```python
from build123d import *

# Parameters (mm, degrees)
SKETCH_1_W               = 15
SKETCH_1_H               = 15
SKETCH_1_W_2             = 6
SKETCH_1_H_2             = 6
SKETCH_1_W_3             = 2
SKETCH_1_H_3             = 2.75
SKETCH_1_W_4             = 2.75
SKETCH_1_H_4             = 2
EXTRUDE_1_DEPTH          = 10
SKETCH_2_W               = 2
SKETCH_2_H               = 4
CUT_EXTRUDE_1_DEPTH      = 2.75
SKETCH_3_W               = 4
SKETCH_3_H               = 2
CUT_EXTRUDE_2_DEPTH      = 2.75
SKETCH_4_W               = 2
SKETCH_4_H               = 4
CUT_EXTRUDE_3_DEPTH      = 2.75
SKETCH_5_W               = 4
SKETCH_5_H               = 2
CUT_EXTRUDE_4_DEPTH      = 2.75
SKETCH_6_W               = 5.5
SKETCH_6_H               = 3
CUT_EXTRUDE_5_DEPTH      = 18.75
SKETCH_7_W               = 3
SKETCH_7_H               = 5.5
CUT_EXTRUDE_6_DEPTH      = 18.75
SKETCH_8_W               = 8
SKETCH_8_H               = 13
CUT_EXTRUDE_7_DEPTH      = 6
CUT_EXTRUDE_7_DEPTH_BACK = 0.75
SKETCH_9_W               = 8
SKETCH_9_H               = 13
CUT_EXTRUDE_8_DEPTH      = 6
SKETCH_10_W              = 8
SKETCH_10_H              = 13
CUT_EXTRUDE_9_DEPTH      = 6


with BuildPart() as part:
    # ｽｹｯﾁ1 → ﾎﾞｽ - 押し出し1 (new body)
    with BuildSketch(Plane.XY):
        with Locations((-13.66786655, 0.754091784)):
            Rectangle(SKETCH_1_W, SKETCH_1_H)
        with Locations((-17.16786655, -2.745908216)):
            Rectangle(SKETCH_1_W_2, SKETCH_1_H_2, mode=Mode.SUBTRACT)
        with Locations((-10.16786655, -2.745908216)):
            Rectangle(SKETCH_1_W_2, SKETCH_1_H_2, mode=Mode.SUBTRACT)
        with Locations((-10.16786655, 4.254091784)):
            Rectangle(SKETCH_1_W_2, SKETCH_1_H_2, mode=Mode.SUBTRACT)
        with Locations((-17.16786655, 4.254091784)):
            Rectangle(SKETCH_1_W_2, SKETCH_1_H_2, mode=Mode.SUBTRACT)
        with Locations((-13.66786655, 9.629091784)):
            Rectangle(SKETCH_1_W_3, SKETCH_1_H_3)
        with Locations((-22.54286655, 0.754091784)):
            Rectangle(SKETCH_1_W_4, SKETCH_1_H_4)
        with Locations((-4.79286655, 0.754091784)):
            Rectangle(SKETCH_1_W_4, SKETCH_1_H_4)
        with Locations((-13.66786655, -8.120908216)):
            Rectangle(SKETCH_1_W_3, SKETCH_1_H_3)
    extrude(amount=EXTRUDE_1_DEPTH)

    # ｽｹｯﾁ2 → ｶｯﾄ - 押し出し1 (cut)
    with BuildSketch(Plane(origin=(0, 11.004091784, 0), x_dir=(1, 0, 0), z_dir=(0, 1, 0))):
        with Locations((-13.66786655, -2)):
            Rectangle(SKETCH_2_W, SKETCH_2_H)
        with Locations((-13.66786655, -8)):
            Rectangle(SKETCH_2_W, SKETCH_2_H)
    extrude(amount=-CUT_EXTRUDE_1_DEPTH, mode=Mode.SUBTRACT)

    # ｽｹｯﾁ3 → ｶｯﾄ - 押し出し2 (cut)
    with BuildSketch(Plane(origin=(-3.41786655, 0, 0), x_dir=(0, 0, -1), z_dir=(1, 0, 0))):
        with Locations((-8, 0.754091784)):
            Rectangle(SKETCH_3_W, SKETCH_3_H)
        with Locations((-2, 0.754091784)):
            Rectangle(SKETCH_3_W, SKETCH_3_H)
    extrude(amount=-CUT_EXTRUDE_2_DEPTH, mode=Mode.SUBTRACT)

    # ｽｹｯﾁ4 → ｶｯﾄ - 押し出し3 (cut)
    with BuildSketch(Plane.XZ.offset(9.495908216)):
        with Locations((-13.66786655, 8)):
            Rectangle(SKETCH_4_W, SKETCH_4_H)
        with Locations((-13.66786655, 2)):
            Rectangle(SKETCH_4_W, SKETCH_4_H)
    extrude(amount=-CUT_EXTRUDE_3_DEPTH, mode=Mode.SUBTRACT)

    # ｽｹｯﾁ5 → ｶｯﾄ - 押し出し4 (cut)
    with BuildSketch(Plane.ZY.offset(23.91786655)):
        with Locations((2, 0.754091784)):
            Rectangle(SKETCH_5_W, SKETCH_5_H)
        with Locations((8, 0.754091784)):
            Rectangle(SKETCH_5_W, SKETCH_5_H)
    extrude(amount=-CUT_EXTRUDE_4_DEPTH, mode=Mode.SUBTRACT)

    # ｽｹｯﾁ6 → ｶｯﾄ - 押し出し5 (cut, through all)
    with BuildSketch(Plane(origin=(0, 8.254091784, 0), x_dir=(1, 0, 0), z_dir=(0, 1, 0))):
        with Locations((-17.41786655, -2.5)):
            Rectangle(SKETCH_6_W, SKETCH_6_H)
        with Locations((-9.91786655, -2.5)):
            Rectangle(SKETCH_6_W, SKETCH_6_H)
        with Locations((-17.41786655, -7.5)):
            Rectangle(SKETCH_6_W, SKETCH_6_H)
        with Locations((-9.91786655, -7.5)):
            Rectangle(SKETCH_6_W, SKETCH_6_H)
    extrude(amount=-CUT_EXTRUDE_5_DEPTH, mode=Mode.SUBTRACT)

    # ｽｹｯﾁ7 → ｶｯﾄ - 押し出し6 (cut, through all)
    with BuildSketch(Plane(origin=(-6.16786655, 0, 0), x_dir=(0, 0, -1), z_dir=(1, 0, 0))):
        with Locations((-7.5, 4.504091784)):
            Rectangle(SKETCH_7_W, SKETCH_7_H)
        with Locations((-2.5, 4.504091784)):
            Rectangle(SKETCH_7_W, SKETCH_7_H)
        with Locations((-7.5, -2.995908216)):
            Rectangle(SKETCH_7_W, SKETCH_7_H)
        with Locations((-2.5, -2.995908216)):
            Rectangle(SKETCH_7_W, SKETCH_7_H)
    extrude(amount=-CUT_EXTRUDE_6_DEPTH, mode=Mode.SUBTRACT)

    # ｽｹｯﾁ8 → ｶｯﾄ - 押し出し7 (cut, two sides)
    with BuildSketch(Plane.ZY.offset(14.16786655)) as cut_extrude_7_sk:
        with Locations((5, 0.754091784)):
            Rectangle(SKETCH_8_W, SKETCH_8_H)
    extrude(amount=CUT_EXTRUDE_7_DEPTH, mode=Mode.SUBTRACT)
    extrude(cut_extrude_7_sk.sketch, amount=-CUT_EXTRUDE_7_DEPTH_BACK, mode=Mode.SUBTRACT)

    # ｽｹｯﾁ9 → ｶｯﾄ - 押し出し8 (cut)
    with BuildSketch(Plane(origin=(-13.16786655, 0, 0), x_dir=(0, 0, -1), z_dir=(1, 0, 0))):
        with Locations((-5, 0.754091784)):
            Rectangle(SKETCH_9_W, SKETCH_9_H)
    extrude(amount=CUT_EXTRUDE_8_DEPTH, mode=Mode.SUBTRACT)

    # ｽｹｯﾁ10 → ｶｯﾄ - 押し出し9 (cut)
    with BuildSketch(Plane(origin=(-13.16786655, 0, 0), x_dir=(0, 0, -1), z_dir=(1, 0, 0))):
        with Locations((-5, 0.754091784)):
            Rectangle(SKETCH_10_W, SKETCH_10_H)
    extrude(amount=-CUT_EXTRUDE_9_DEPTH, mode=Mode.SUBTRACT)


solid = part.part
```
Check sheet for the modelled part. Datum: model origin and axes. Units: mm. A direction names the side the tool comes from. Round coordinates to 2 decimals unless told otherwise and drop trailing zeros. Order: outer loops, then holes, each group sorted by start corner. A loop starts at its lowest first (then second) coordinate and runs counter-clockwise, first axis right, second up.
1) Mould release check, pull along Z, two halves, no side actions. Record for faces 4 (the flat face through (-17.2, 0.254, 9.5)), 5 (the flat face through (-21, -0.246, 3)), 6 (the flat face through (-23, 1, 6)): +Z half, -Z half, draft (parallel to the pull), parting line (faces both ways), or undercut.
2) Section check A-A (x = -19.5). Give the number of separate pieces and of enclosed holes in the cut face, and give its area (3 significant figures).
3) Section check B-B (z = 9.5). Record the boundary of the cut face in (x, y), and give its area (3 significant figures).
4) Go/stop test with flat-tipped pins: pin 1 Ø2 at (x, z) = (-14, 8) entering from -Y; pin 2 Ø1.5 at (y, z) = (-4, 6) entering from -X; pin 3 Ø1 at (x, y) = (-13.5, 9) entering from +Z. Record where each tip stops, or that it passes through.
5) Scan lines: line 1 (X direction, y = 2.25, z = 0.5); line 2 (Y direction, x = -9, z = 9.5); line 3 (X direction, y = -6.5, z = 2.5). Record each from-to range of solid material in increasing order.
6) Tool access check on faces 1 (the flat face through (-14.668, 10, 5)), 2 (the flat face through (-12.668, 8, 3)), 3 (the flat face through (-21, 7.254, 8)). Record the directions out of +Z, -Z, +X, -X, +Y, -Y that give a thin tool (end or side, any length) a straight path to the whole face; none if there is none.
7) Section check D-D (y = 9). Record the boundary of the cut face in (x, z).
Result:
1. face 4: draft
1. face 5: undercut
1. face 6: +Z half
2. separate pieces: 8
2. enclosed holes: 0
2. area: 10.0 mm2
3. outline: (-21.17, -6.75) - (-6.17, -6.75) - (-6.17, 8.25) - (-21.17, 8.25) - close; hole (-20.17, -5.75) - (-14.17, -5.75) - (-14.17, 0.25) - (-20.17, 0.25) - close; hole (-20.17, 1.25) - (-14.17, 1.25) - (-14.17, 7.25) - (-20.17, 7.25) - close; hole (-13.17, -5.75) - (-7.17, -5.75) - (-7.17, 0.25) - (-13.17, 0.25) - close; hole (-13.17, 1.25) - (-7.17, 1.25) - (-7.17, 7.25) - (-13.17, 7.25) - close
3. area: 81.0 mm2
4. pin 1: stops at y = -6.75
4. pin 2: stops at x = -21.17
4. pin 3: stops at z = 6
5. line 1: x = -21.17 to -20.17, -14.17 to -13.17, -7.17 to -6.17
5. line 2: y = -6.75 to -5.75, 0.25 to 1.25, 7.25 to 8.25
5. line 3: x = -21.17 to -20.17, -14.67 to -12.67, -7.17 to -6.17
6. face 1: +Z, -Z, -X, +Y
6. face 2: +Y, -Y
6. face 3: +X, -X
7. outline: (-14.67, 4) - (-12.67, 4) - (-12.67, 6) - (-14.67, 6) - close
